Source: CAD feature listing. Evaluate the final solid. Frame: model axes, mm. A direction names the side the tool comes from. Round coordinates to 2 decimals unless told otherwise and drop trailing zeros. Write each loop counter-clockwise with the first axis right and the second up, starting at its lowest first coordinate (ties: lowest second). Pieces come first, ordered by that corner, then holes. Notation, with made-up numbers: M 70.25,63.5 L 86.25,63.5 A24 ccw 86.25,99.5 Z; hole C 74,24.5 d10. An arc over 180 degrees is marked long. Answer in a Markdown table with one row per item. Add a question column.
Item 1: Material intervals for probe 1 along Y at (x, z) = (0.75, -0.8); probe 2 along X at (y, z) = (-11, -0.25); probe 3 along Z at (x, y) = (0.2, -34), sorted ascending.
Item 2: Contact query for flat-ended pins moving along their axis: pin 1 (1 mm diameter, centred on y = -14.5, z = -0.5, fed in from -X); pin 2 (1 mm diameter, centred on x = -0.5, y = -22, fed in from -Z). Output: stop coordinate, or through.
Item 3: Cut plane A-A on y = -3.5. Return loops of the section in (x, z), and give its area (3 significant figures).
Item 4: Set-up query: faces 1 (the face through (0.464, -38.27, -0.007)), 2 (the face through (0.225, -18.744, 0.715)). Return all of +Z, -Z, +X, -X, +Y, -Y with unobstructed straight access to the full face (end or side cutting, diameter ignored); none if empty.
from build123d import *

# Parameters (mm, degrees)
SKETCH_1_R               = 0.75
EXTRUDE_1_DEPTH          = 40
SKETCH_2_R               = 1.5
EXTRUDE_2_DEPTH          = 1
CUT_EXTRUDE_2_DEPTH      = 41.056210505
CUT_EXTRUDE_2_DEPTH_BACK = 41.056210505
CUT_EXTRUDE_3_DEPTH      = 41.056210505
CUT_EXTRUDE_3_DEPTH_BACK = 41.056210505


with BuildPart() as part:
    # Эскиз1 → Бобышка-Вытянуть1 (new body)
    with BuildSketch(Plane(origin=(0, 0, 0), x_dir=(1, 0, 0), z_dir=(0, 1, 0))):
        with Locations(Location((0, 0, 0), (0, 0, 270))):
            Circle(SKETCH_1_R)
    extrude(amount=-EXTRUDE_1_DEPTH)

    # Эскиз2 → Бобышка-Вытянуть2 (add)
    with BuildSketch(Plane(origin=(0, 0, 0), x_dir=(1, 0, 0), z_dir=(0, 1, 0))):
        with Locations(Location((0, 0, 0), (0, 0, 270))):
            Circle(SKETCH_2_R)
    extrude(amount=EXTRUDE_2_DEPTH)

    # Эскиз5 → Вырез-Вытянуть2 (cut, two sides: drawn at the far end of the back side and taken through both)
    with BuildSketch(Plane(origin=(0, 0, 0), x_dir=(0, 0, -1), z_dir=(1, 0, 0)).offset(-CUT_EXTRUDE_2_DEPTH_BACK)):
        Polygon((-1.201318644, -35.516617784), (-1.201318644, -40.516617784), (1.201318644, -40.516617784), (1.201318644, -35.516617784), (0, -40), align=None)
    extrude(amount=CUT_EXTRUDE_2_DEPTH + CUT_EXTRUDE_2_DEPTH_BACK, mode=Mode.SUBTRACT)

    # Эскиз7 → Вырез-Вытянуть3 (cut, two sides: drawn at the far end of the back side and taken through both)
    with BuildSketch(Plane.XY.offset(-CUT_EXTRUDE_3_DEPTH_BACK)):
        Polygon((-1.267511878, -35.269581272), (-1.267511878, -40.269581272), (1.267511878, -40.269581272), (1.267511878, -35.269581272), (0, -40), align=None)
    extrude(amount=CUT_EXTRUDE_3_DEPTH + CUT_EXTRUDE_3_DEPTH_BACK, mode=Mode.SUBTRACT)


solid = part.part
Results below:
| question | item | result |
|---|---|---|
| 1 | probe 1 | 0 to 1 |
| 1 | probe 2 | -0.71 to 0.71 |
| 1 | probe 3 | -0.72 to 0.72 |
| 2 | pin 1 | x = -0.75 |
| 2 | pin 2 | z = -0.75 |
| 3 | outline | C 0,0 d1.5 |
| 3 | area | 1.77 mm2 |
| 4 | face 1 | +Z, -Z, +X, -Y |
| 4 | face 2 | -Y |
